from build123d import *

# Parameters (mm, degrees)
SKETCH_1_R               = 1.05
SKETCH_1_R_2             = 1.55
SKETCH_1_R_3             = 1.75
EXTRUDE_1_DEPTH          = 3
CUT_EXTRUDE_1_DEPTH      = 10
SKETCH_5_W               = 12.2
SKETCH_5_H               = 4.62
CUT_EXTRUDE_3_DEPTH      = 1
CUT_EXTRUDE_3_DEPTH_BACK = 1.22


with BuildPart() as part:
    # 草图1 → 凸台-拉伸1 (new body)
    with BuildSketch(Plane(origin=(0, 0, 0), x_dir=(1, 0, 0), z_dir=(0, 1, 0))):
        with BuildLine():
            Line((0, 43), (0, 0))
            Line((0, 0), (62, 0))
            Line((62, 0), (62, 43))
            Line((62, 43), (54, 43))
            ThreePointArc((54, 43), (47, 50), (40, 43))
            Line((40, 43), (22, 43))
            ThreePointArc((22, 43), (15, 50), (8, 43))
            Line((8, 43), (0, 43))
        make_face()
        with Locations((3, 3)):
            Circle(SKETCH_1_R, mode=Mode.SUBTRACT)
        with Locations((15, 10)):
            Circle(SKETCH_1_R_2, mode=Mode.SUBTRACT)
        with Locations((31, 3)):
            Circle(SKETCH_1_R, mode=Mode.SUBTRACT)
        with Locations((59, 3)):
            Circle(SKETCH_1_R, mode=Mode.SUBTRACT)
        with Locations((47, 10)):
            Circle(SKETCH_1_R_2, mode=Mode.SUBTRACT)
        with Locations((31, 23.5)):
            Circle(SKETCH_1_R, mode=Mode.SUBTRACT)
        with Locations((3, 40)):
            Circle(SKETCH_1_R, mode=Mode.SUBTRACT)
        with Locations((15, 37.8)):
            Circle(SKETCH_1_R, mode=Mode.SUBTRACT)
        with Locations((21.9, 40)):
            Circle(SKETCH_1_R, mode=Mode.SUBTRACT)
        with Locations((40.1, 40)):
            Circle(SKETCH_1_R, mode=Mode.SUBTRACT)
        with Locations((47, 37.8)):
            Circle(SKETCH_1_R, mode=Mode.SUBTRACT)
        with Locations((59, 40)):
            Circle(SKETCH_1_R, mode=Mode.SUBTRACT)
        with Locations((15, 45)):
            Circle(SKETCH_1_R_3, mode=Mode.SUBTRACT)
        with Locations((47, 45)):
            Circle(SKETCH_1_R_3, mode=Mode.SUBTRACT)
    extrude(amount=EXTRUDE_1_DEPTH)

    # 草图2 → 切除-拉伸1 (cut)
    with BuildSketch(Plane(origin=(0, 3, 0), x_dir=(1, 0, 0), z_dir=(0, 1, 0))):
        Polygon((31, 43), (37.1, 43), (37.1, 26.05), (24.9, 26.05), (24.9, 43), align=None)
    extrude(amount=-CUT_EXTRUDE_1_DEPTH, mode=Mode.SUBTRACT)

    # 草图5 → 切除-拉伸3 (cut, two sides)
    with BuildSketch(Plane(origin=(0, 3, 0), x_dir=(1, 0, 0), z_dir=(0, 1, 0))) as cut_extrude_3_sk:
        with Locations((31, 23.74)):
            Rectangle(SKETCH_5_W, SKETCH_5_H)
    extrude(amount=CUT_EXTRUDE_3_DEPTH, mode=Mode.SUBTRACT)
    extrude(cut_extrude_3_sk.sketch, amount=-CUT_EXTRUDE_3_DEPTH_BACK, mode=Mode.SUBTRACT)


solid = part.part
Model file for the job. Use its own axes, mm. A direction names the side the tool comes from. Round coordinates to 2 decimals unless told otherwise and drop trailing zeros. Order: outer loops, then holes, each group sorted by start corner. A loop starts at its lowest first (then second) coordinate and runs counter-clockwise, first axis right, second up.
(1) Band-saw the part on D-D (z = -37.8). List the corners of the cut face in (x, y), then the cut area to 3 significant figures.
(2) Pin check, flat tips, straight feed: pin 1 (1.4 mm diameter, centred on x = 23, y = 2, fed in from -Z); pin 2 (1.4 mm diameter, centred on x = 33, y = 0.5, fed in from -Z). Stop position of each tip, or through.
(3) Pull direction X, two halves, no side cores. Call faces 4 (the face through (0, 1, -22)), 5 (the face through (62, 1, -21)), 6 (the face through (48.617, 1.479, -44.33)), 7 (the face through (4, 1, -43)): released by +X, released by -X, zero draft, split by the parting line, or undercut.
(4) Band-saw the part on B-B (z = -23.5). List the corners of the cut face in (x, y), then the cut area to 3 significant figures.
(5) Band-saw the part on C-C (x = 15). List the corners of the cut face in (y, z), then the cut area to 3 significant figures.
(6) 3-axis set-ups, long thin cutter, end or side, ignore diameter. For faces 1 (the face through (31, 2, -21.43)), 2 (the face through (60, 1.48, -3.32)), 3 (the face through (39, 1, -43)): which of +Z, -Z, +X, -X, +Y, -Y reach the whole face in a straight line?
(7) Drill centre lines: line 1 (X direction, y = 0.7, z = -40); line 2 (Z direction, x = 3, y = 0.6); line 3 (Z direction, x = 15, y = 2.2). Where is each one in solid material? Low to high.
(8) Band-saw the part on A-A (x = 59). List the corners of the cut face in (y, z), then the cut area to 3 significant figures.
Verdict:
1. outline: (0, 0) - (13.95, 0) - (13.95, 3) - (0, 3) - close; (16.05, 0) - (24.9, 0) - (24.9, 3) - (16.05, 3) - close; (37.1, 0) - (45.95, 0) - (45.95, 3) - (37.1, 3) - close; (48.05, 0) - (62, 0) - (62, 3) - (48.05, 3) - close
1. area: 137 mm2
2. pin 1: stops at z = -43
2. pin 2: stops at z = -26.05
3. face 4: released by -X
3. face 5: released by +X
3. face 6: undercut
3. face 7: zero draft
4. outline: (0, 0) - (29.95, 0) - (29.95, 1.78) - (24.9, 1.78) - (24.9, 3) - (0, 3) - close; (32.05, 0) - (62, 0) - (62, 3) - (37.1, 3) - (37.1, 1.78) - (32.05, 1.78) - close
4. area: 167 mm2
5. outline: (0, -50) - (3, -50) - (3, -46.75) - (0, -46.75) - close; (0, -43.25) - (3, -43.25) - (3, -38.85) - (0, -38.85) - close; (0, -36.75) - (3, -36.75) - (3, -11.55) - (0, -11.55) - close; (0, -8.45) - (3, -8.45) - (3, 0) - (0, 0) - close
5. area: 124 mm2
6. face 1: -Z, +Y
6. face 2: +Y, -Y
6. face 3: -Z, +Y, -Y
7. line 1: x = 0 to 1.95, 4.05 to 20.85, 22.95 to 24.9, 37.1 to 39.05, 41.15 to 57.95, 60.05 to 62
7. line 2: z = -43 to -41.05, -38.95 to -4.05, -1.95 to 0
7. line 3: z = -50 to -46.75, -43.25 to -38.85, -36.75 to -11.55, -8.45 to 0
8. outline: (0, -43) - (3, -43) - (3, -41.05) - (0, -41.05) - close; (0, -38.95) - (3, -38.95) - (3, -4.05) - (0, -4.05) - close; (0, -1.95) - (3, -1.95) - (3, 0) - (0, 0) - close
8. area: 116 mm2
